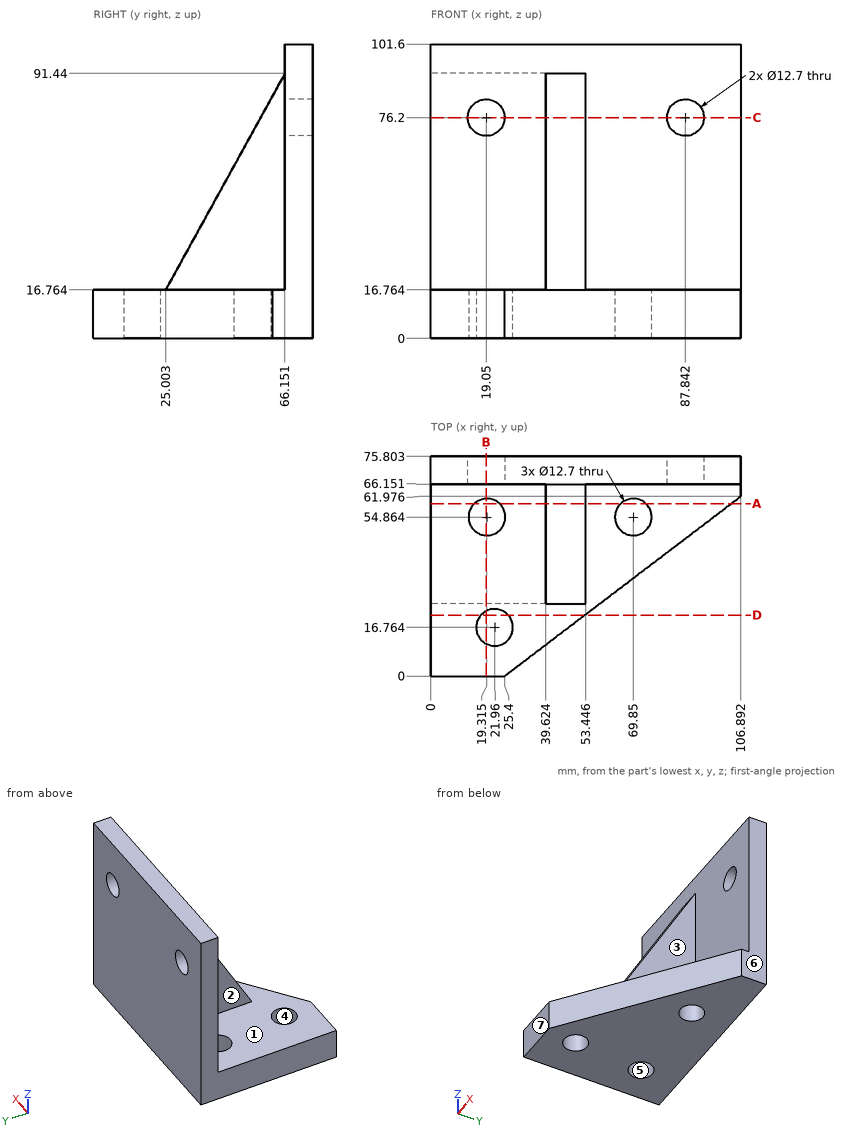
Study the drawing (mm; zero at the part's minimum x, y, z) and answer. A direction names the side the tool comes from. Give positions to 0.01 mm unless a question says otherwise; leave off trailing zeros. Order: outer loops, then holes, each group sorted by start corner. A loop starts at its lowest first (then second) coordinate and runs counter-clockwise, first axis right, second up. Notation, with made-up numbers: M 40.5,-9.5 L 60.5,-9.5 A21 ccw 60.5,5.5 Z; hole C 27,-16.5 d4. An arc over 180 degrees is marked long. Put each result on its own line as item: value. Start each with the question number.
Item 1: Flat-ended cylindrical pins translate along their axes: P1, Ø16.5, axis at x = 21.96, y = 16.76, coming from the +Z side; P2, Ø16.5, axis at x = 19.05, z = 76.2, coming from the -Y side; P3, Ø7.5, axis at x = 87.84, z = 76.2, coming from the +Y side; P4, Ø12, axis at x = 57, y = 38.5, coming from the +Z side. Find the tip coordinate at first contact, or state that the pin passes through.
Item 2: Which of the six approach directions +Z, -Z, +X, -X, +Y, -Y give full straight-line access (tool end or side, diameter ignored) to the marked faces 1, 2 and 3?
Item 3: For a pull along Y with two mould halves and no side action, classify the marked faces 4, 5, 6 and 7 as +Y half, -Y half, draft (parallel to the pull), parting line (faces both ways), or undercut.
Item 4: Find the intervals of material crossed by line 1 along Z through (x, y) = (19, 71); line 2 along X through (y, z) = (70, 76) (1 decimal); line 3 along Z through (x, y) = (33.5, 48), in increasing order.
Item 5: The part is cut by section A-A, the plane y = 59.5. Determine the outline of the cut face in (x, z) (1 decimal).
Item 6: The part is cut by section C-C, the plane z = 76.2. Determine the outline of the cut face in (x, y) (1 decimal).
Item 7: The part is cut by section B-B, the plane x = 19.05. Determine the outline of the cut face in (y, z), and give its area (4 significant figures).
Item 8: The part is cut by section D-D, the plane y = 21. Determine the outline of the cut face in (x, z).
Answer key:
1. P1: stops at z = 16.76
1. P2: stops at y = 66.15
1. P3: passes through
1. P4: stops at z = 50.03
2. face 1: +Z, -Y
2. face 2: +Z, -X, -Y
2. face 3: +Z, +X, -Y
3. face 4: undercut
3. face 5: undercut
3. face 6: draft
3. face 7: -Y half
4. line 1: z = 0 to 69.85, 82.55 to 101.6
4. line 2: x = 0 to 12.7, 25.4 to 81.5, 94.2 to 106.9
4. line 3: z = 0 to 16.76
5. outline: M 0,0 L 15,0 L 15,16.8 L 0,16.8 Z; M 23.7,0 L 65.5,0 L 65.5,16.8 L 53.4,16.8 L 53.4,79.4 L 39.6,79.4 L 39.6,16.8 L 23.7,16.8 Z; M 74.2,0 L 103.6,0 L 103.6,16.8 L 74.2,16.8 Z
6. outline: M 0,66.2 L 12.7,66.2 L 12.7,75.8 L 0,75.8 Z; M 25.4,66.2 L 39.6,66.2 L 39.6,57.8 L 53.4,57.8 L 53.4,66.2 L 81.5,66.2 L 81.5,75.8 L 25.4,75.8 Z; M 94.2,66.2 L 106.9,66.2 L 106.9,75.8 L 94.2,75.8 Z
7. outline: M 0,0 L 11.12,0 L 11.12,16.76 L 0,16.76 Z; M 22.41,0 L 48.52,0 L 48.52,16.76 L 22.41,16.76 Z; M 61.21,0 L 75.8,0 L 75.8,69.85 L 66.15,69.85 L 66.15,16.76 L 61.21,16.76 Z; M 66.15,82.55 L 75.8,82.55 L 75.8,101.6 L 66.15,101.6 Z
7. area: 1,565 mm²
8. outline: M 0,0 L 17.23,0 L 17.23,16.76 L 0,16.76 Z; M 26.69,0 L 53.01,0 L 53.01,16.76 L 26.69,16.76 Z
